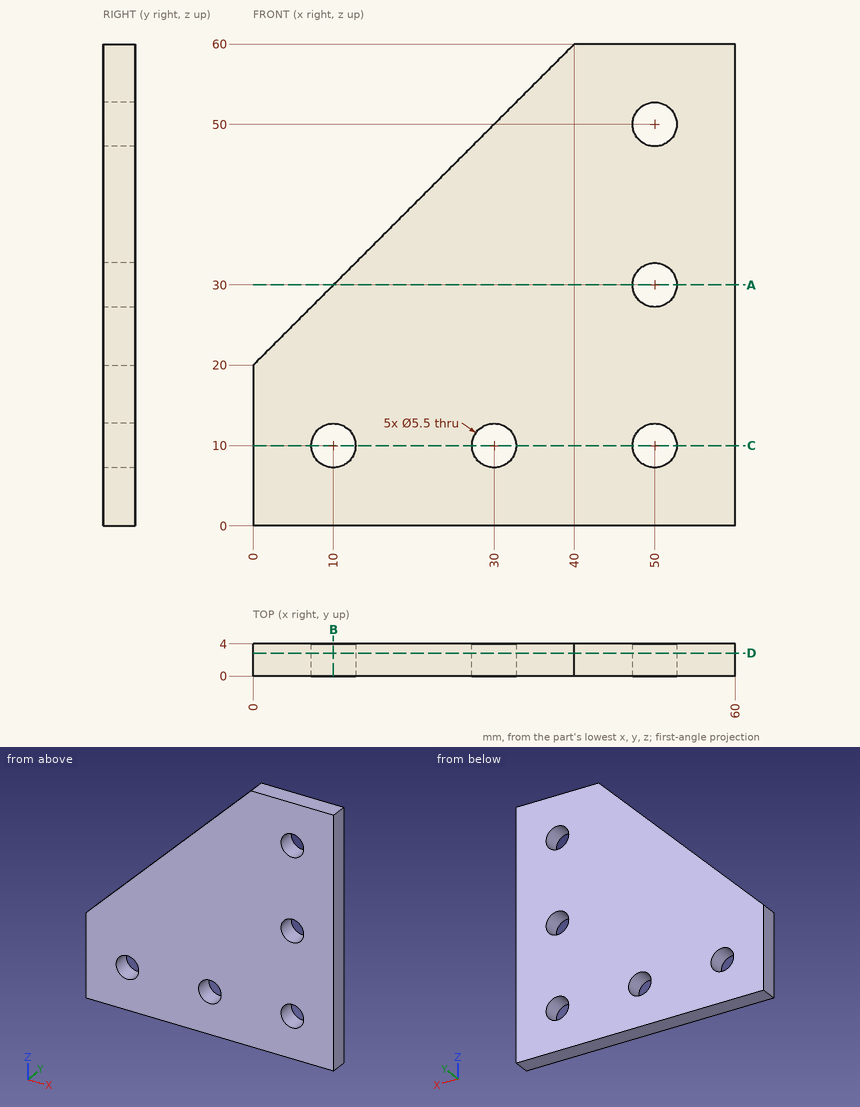
Design review of the part shown in the three views and the two pictorial views. Dimensions are in mm from the part's minimum x, y and z. Round coordinates to 2 decimals unless told otherwise and drop trailing zeros. Order: outer loops, then holes, each group sorted by start corner. A loop starts at its lowest first (then second) coordinate and runs counter-clockwise, first axis right, second up. Notation, with made-up numbers: (60.25, 88) - (76.25, 88) arc R21 cw to (76.25, 100) - close; hole circle Ø10 at (80, -16.5). An arc over 180 degrees is marked (long way). Answer in a Markdown table with one row per item.
(1) Take a section at A-A on z = 30. Write out the cut boundary in (x, y).
Result set:
| item | result |
|---|---|
| outline | (10, 0) - (47.25, 0) - (47.25, 4) - (10, 4) - close; (52.75, 0) - (60, 0) - (60, 4) - (52.75, 4) - close |
(2) For line 1 (Z direction, x = 50, y = 3.25); line 2 (X direction, y = 3.85, z = 40); line 3 (Z direction, x = 30, y = 3.5), list the stretches that pass through material, from the lowest coordinate up. Write a range as from..to.
Result set:
| item | result |
|---|---|
| line 1 | z = 0..7.25, 12.75..27.25, 32.75..47.25, 52.75..60 |
| line 2 | x = 20..60 |
| line 3 | z = 0..7.25, 12.75..50 |
(3) Take a section at D-D on y = 2.85. Write out the cut boundary in (x, z).
Result set:
| item | result |
|---|---|
| outline | (0, 0) - (60, 0) - (60, 60) - (40, 60) - (0, 20) - close; hole circle Ø5.5 at (10, 10); hole circle Ø5.5 at (30, 10); hole circle Ø5.5 at (50, 10); hole circle Ø5.5 at (50, 30); hole circle Ø5.5 at (50, 50) |
(4) Take a section at B-B on x = 10. Write out the cut boundary in (y, z).
Result set:
| item | result |
|---|---|
| outline | (0, 0) - (4, 0) - (4, 7.25) - (0, 7.25) - close; (0, 12.75) - (4, 12.75) - (4, 30) - (0, 30) - close |
(5) Take a section at C-C on z = 10. Write out the cut boundary in (x, y).
Result set:
| item | result |
|---|---|
| outline | (0, 0) - (7.25, 0) - (7.25, 4) - (0, 4) - close; (12.75, 0) - (27.25, 0) - (27.25, 4) - (12.75, 4) - close; (32.75, 0) - (47.25, 0) - (47.25, 4) - (32.75, 4) - close; (52.75, 0) - (60, 0) - (60, 4) - (52.75, 4) - close |
